Geometry check sheet. Reference: the model listing, model coordinates, mm. Coordinates: 2 decimals unless noted, no trailing zeros. Loops run counter-clockwise (first coordinate to the right, second up) from the corner with the lowest first, then second, coordinate; pieces in that order, holes last. Notation, with made-up numbers: M -16.5,12 L 30.5,12 A15 cw 30.5,20 Z; hole C 80.25,66.25 d4. An arc over 180 degrees is marked long. One line per question, with ' | ' between items. Start each with the question number.
Autodesk Inventor part; units mm, degrees
ref_plane "YZ Plane" through (0, 0, 0) normal (1, 0, 0) x (0, 1, 0)
ref_plane "XZ Plane" through (0, 0, 0) normal (0, 1, 0) x (-1, 0, 0)
ref_plane "XY Plane" through (0, 0, 0) normal (0, 0, 1) x (1, 0, 0)
sketch "Sketch1" plane through (0, 0, 0) normal (0, 1, 0) x (-1, 0, 0)
  line L0 (25.4, 47.498) -> (-25.4, 47.498)
  line L1 (-25.4, 47.498) -> (-25.4, -47.498)
  line L2 (-25.4, -47.498) -> (25.4, -47.498)
  line L3 (25.4, -47.498) -> (25.4, 47.498)
  line L4 (25.4, 47.498) -> (-25.4, -47.498) construction
  line L5 (-25.4, 47.498) -> (25.4, -47.498) construction
  point P0 (0, 0)
  dimension "d0" = 50.8
  dimension "d1" = 94.996
extrude "Extrusion1" add sketch "Sketch1" along normal blind 6.35
sketch "Sketch2" plane through (25.4, 0, 47.498) normal (1, 0, 0) x (0, 0, -1)
  line L0 (-35.052, 19.05) -> (130.048, 19.05)
  line L1 (130.048, 19.05) -> (130.048, 0)
  line L2 (130.048, 0) -> (-35.052, 0)
  line L3 (-35.052, 0) -> (-35.052, 19.05)
  line L4 (-35.052, 19.05) -> (130.048, 0) construction
  line L5 (130.048, 19.05) -> (-35.052, 0) construction
  line L6 (0, 0) -> (94.996, 0)
  circle A0 centre (-35.052, 9.525) radius 9.525
  circle A1 centre (130.048, 9.525) radius 9.525
  point P0 (47.498, 0)
  point P1 (47.498, 9.525)
  point P2 (47.498, 0)
  dimension "d4" = 165.1
  dimension "d5" = 19.05
extrude "Extrusion2" add sketch "Sketch2" against normal blind 6.35
fillet "Fillet1" radius 2.54 9 edges at (19.05, 0, -65.024) (19.05, 19.05, 0) (19.05, 9.525, 92.075) (19.05, 0, 65.024) (19.05, 9.525, -92.075) (25.4, 19.05, 0) (25.4, 9.525, 92.075) (25.4, 0, 0) (25.4, 9.525, -92.075)
mirror "Mirror1" about plane through (0, 0, 0) normal (1, 0, 0) of "Extrusion2", "Fillet1"
sketch "Sketch3" plane through (25.4, 9.525, 82.55) normal (1, 0, 0) x (0, 0, -1)
  arc A0 (165.1, -6.985) -> (165.1, 6.985) centre (165.1, 0) ccw
  point P0 (82.55, -9.525)
  point P1 (0, 0)
hole "Hole1" at (25.4, 9.525, 82.55) at (25.4, 9.525, -82.55) direction (-1, 0, 0) diameter 8.89 end through all
properties part number "Thick Leg"
1. Sectioned sample at B-B (z = -38.5). Record the cut outline in (x, y), and give its area (3 significant figures).
2. Thickness scan on line 1 (Y direction, x = -21.25, z = -82.55); line 2 (X direction, y = 10.5, z = -19.5); line 3 (Y direction, x = 23, z = 82). Record the ranges inside material, lowest first.
3. Draft check along Y on faces 1 (the cylindrical face through (22.181, 11.227, -86.656)), 2 (the flat face through (-25.4, 9, -1)), 3 (the flat face through (0, 6.35, 1)), 4 (the flat face through (0, 0, 1)). Enter one of: +Y half, -Y half, draft (parallel to the pull), parting line (faces both ways), or undercut.
4. Depth check by flat-ended pin: pin 1 Ø7 at (y, z) = (9.525, -82.55) entering from -X; pin 2 Ø8 at (x, y) = (-11, 9.5) entering from -Z; pin 3 Ø8 at (x, z) = (-8, -36) entering from +Y; pin 4 Ø7 at (x, y) = (-10.5, 1.5) entering from +Z. Enter the tip coordinate at first touch or a pass-through.
5. Sectioned sample at A-A (z = 55). Record the cut outline in (x, y).
6. Sectioned sample at C-C (x = 15). Record the cut outline in (y, z), and give its area (3 significant figures).
Result:
1) outline: M -25.4,2.54 A2.54 ccw -22.86,0 L 22.86,0 A2.54 ccw 25.4,2.54 L 25.4,16.51 A2.54 ccw 22.86,19.05 L 21.59,19.05 A2.54 ccw 19.05,16.51 L 19.05,6.35 L -19.05,6.35 L -19.05,16.51 A2.54 ccw -21.59,19.05 L -22.86,19.05 A2.54 ccw -25.4,16.51 Z | area: 476 mm2
2) line 1: y = 0.02 to 5.08, 13.97 to 19.03 | line 2: x = -25.4 to -19.05, 19.05 to 25.4 | line 3: y = 0 to 5.11, 13.94 to 19.05
3) face 1: undercut | face 2: draft | face 3: +Y half | face 4: -Y half
4) pin 1: passes through | pin 2: stops at z = -47.5 | pin 3: stops at y = 6.35 | pin 4: stops at z = 47.5
5) outline: M -25.4,2.54 A2.54 ccw -22.86,0 L -21.59,0 A2.54 ccw -19.05,2.54 L -19.05,16.51 A2.54 ccw -21.59,19.05 L -22.86,19.05 A2.54 ccw -25.4,16.51 Z; M 19.05,2.54 A2.54 ccw 21.59,0 L 22.86,0 A2.54 ccw 25.4,2.54 L 25.4,16.51 A2.54 ccw 22.86,19.05 L 21.59,19.05 A2.54 ccw 19.05,16.51 Z
6) outline: M 0,-47.5 L 6.35,-47.5 L 6.35,47.5 L 0,47.5 Z | area: 603 mm2
